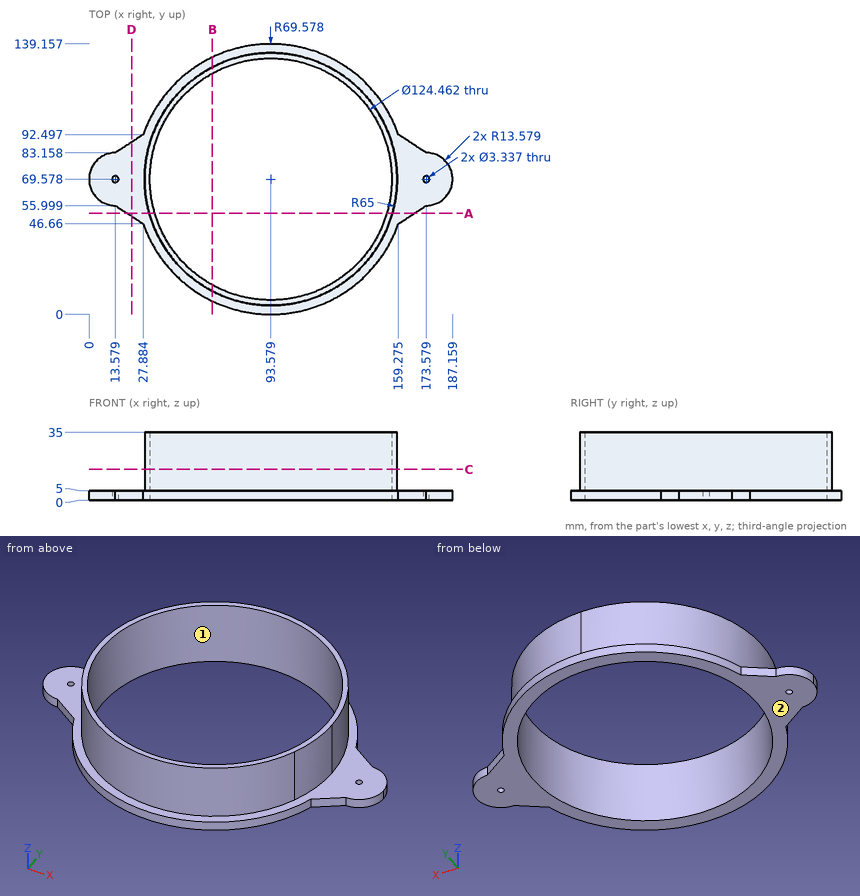
Here's the drawing with two shaded views (mm, measured from the low corner). I have some questions. Give positions to 0.01 mm unless a question says otherwise; leave off trailing zeros. Order: outer loops, then holes, each group sorted by start corner. A loop starts at its lowest first (then second) coordinate and runs counter-clockwise, first axis right, second up. Notation, with made-up numbers: (40, -23.5) - (80, -23.5) arc R19 ccw to (80, -0.5) - close; hole circle Ø11 at (42, 82). An arc over 180 degrees is marked (long way). Use a Markdown table: item, result. Add a question column.
Q1. If we mould it in two halves opening along Y, with no side actions, what happens to the marked faces 1 and 2? For each: released by +Y, released by -Y, zero draft, split by the parting line, or undercut.
Q2. Please list where these lines run through material, in increasing order: line 1 along Y through (x, z) = (94, 10.5); line 2 along Z through (x, y) = (126, 127); line 3 along X through (y, z) = (96.5, 32) (1 decimal).
Q3. If we section it at B-B on x = 63.5: Write out the boundary of the cut face in (y, z), plus the area to 3 significant figures.
Q4. If we section it at D-D on x = 22: Write out the boundary of the cut face in (y, z) (1 decimal), plus the area to 3 significant figures.
Q5. If we section it at C-C on z = 16: Write out the boundary of the cut face in (x, y), plus the area to 3 significant figures.
Q6. If we section it at A-A on y = 52: Write out the boundary of the cut face in (x, z) (1 decimal).
Q7. I'm going to push flat-ended pins straight in: pin 1 (12 mm diameter, centred on x = 128, z = 10.5, fed in from -Y) (1 decimal); pin 2 (10 mm diameter, centred on x = 96.5, z = 31, fed in from +Y); pin 3 (1.5 mm diameter, centred on x = 152.5, z = 18, fed in from +Y). Where does each tip first touch, or does it pass through?
Answers follow:
| question | item | result |
|---|---|---|
| 1 | face 1 | undercut |
| 1 | face 2 | zero draft |
| 2 | line 1 | y = 4.58 to 7.35, 131.81 to 134.58 |
| 2 | line 2 | z = 0 to 5 |
| 2 | line 3 | x = 34.4 to 37.5, 149.7 to 152.7 |
| 3 | outline | (6.84, 0) - (15.1, 0) - (15.1, 35) - (11.96, 35) - (11.96, 5) - (6.84, 5) - close; (124.06, 0) - (132.32, 0) - (132.32, 5) - (127.2, 5) - (127.2, 35) - (124.06, 35) - close |
| 3 | area | 271 mm^2 |
| 4 | outline | (50.5, 0) - (88.7, 0) - (88.7, 5) - (50.5, 5) - close |
| 4 | area | 191 mm^2 |
| 5 | outline | circle Ø130 at (93.58, 69.58); hole circle Ø124.46 at (93.58, 69.58) |
| 5 | area | 1,110 mm^2 |
| 6 | outline | (19.7, 0) - (33.9, 0) - (33.9, 35) - (31, 35) - (31, 5) - (19.7, 5) - close; (153.3, 0) - (167.5, 0) - (167.5, 5) - (156.2, 5) - (156.2, 35) - (153.3, 35) - close |
| 7 | pin 1 | stops at y = 7.8 |
| 7 | pin 2 | stops at y = 134.58 |
| 7 | pin 3 | stops at y = 98.58 |
